Can you work these out from the drawing? Everything is in mm from the part's minimum corner. A direction names the side the tool comes from. Round coordinates to 2 decimals unless told otherwise and drop trailing zeros. Loops run counter-clockwise (first coordinate to the right, second up) from the corner with the lowest first, then second, coordinate; pieces in that order, holes last. Notation, with made-up numbers: M 15,86 L 51,86 A22 cw 51,104 Z; hole C 52,17.5 d3. An arc over 180 degrees is marked long. Answer in a Markdown table with one row per item.
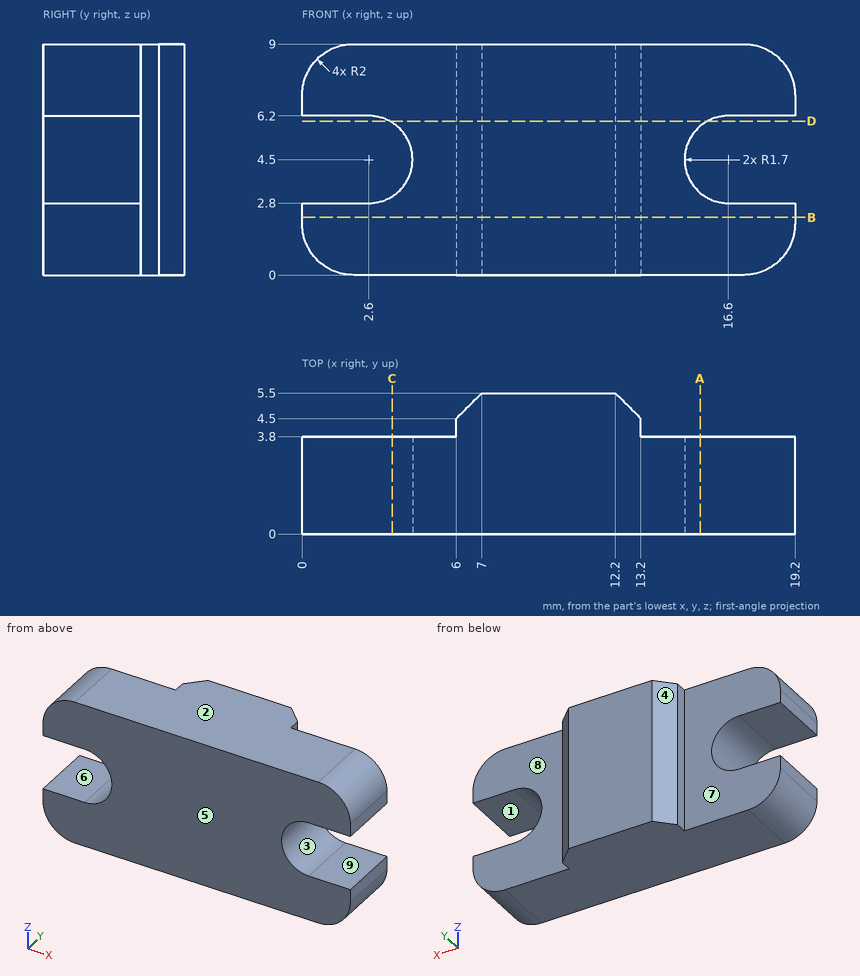
1) Will these pins go through, and if not, where does the flat tip stop? P1, Ø1, axis at x = 6, z = 7, coming from the +Y side; P2, Ø3, axis at x = 18, y = 1, coming from the -Z side; P3, Ø5, axis at x = 2.5, z = 4.5, coming from the +Y side; P4, Ø0.6, axis at y = 4, z = 4.5, coming from the +X side.
Computed:
| item | result |
|---|---|
| P1 | stops at y = 5 |
| P2 | stops at z = 0 |
| P3 | stops at y = 3.8 |
| P4 | stops at x = 14.91 |
2) I want a section at A-A, the plane x = 15.5. Please give me the cut outline in (y, z).
Computed:
| item | result |
|---|---|
| outline | M 0,0 L 3.8,0 L 3.8,3.2 L 0,3.2 Z; M 0,5.8 L 3.8,5.8 L 3.8,9 L 0,9 Z |
3) If we mould it in two halves opening along Z, with no side actions, what happens to the marked faces 1, 2, 3 and 4? For each: released by +Z, released by -Z, zero draft, split by the parting line, or undercut.
Computed:
| item | result |
|---|---|
| face 1 | undercut |
| face 2 | released by +Z |
| face 3 | undercut |
| face 4 | zero draft |
4) I want a section at B-B, the plane z = 2.25. Please give me the cut outline in (x, y).
Computed:
| item | result |
|---|---|
| outline | M 0,0 L 19.2,0 L 19.2,3.8 L 13.2,3.8 L 13.2,4.5 L 12.2,5.5 L 7,5.5 L 6,4.5 L 6,3.8 L 0,3.8 Z |
5) I need wall thicknesses on line 1 (Z direction, x = 2, y = 0.6); line 2 (X direction, y = 1.15, z = 4.5); line 3 (Y direction, x = 18.5, z = 1.5). Which ranges of each line are inside material? Lowest first, please.
Computed:
| item | result |
|---|---|
| line 1 | z = 0 to 2.8, 6.2 to 9 |
| line 2 | x = 4.3 to 14.9 |
| line 3 | y = 0 to 3.8 |
6) I want a section at C-C, the plane x = 3.5. Please give me the cut outline in (y, z).
Computed:
| item | result |
|---|---|
| outline | M 0,0 L 3.8,0 L 3.8,3.06 L 0,3.06 Z; M 0,5.94 L 3.8,5.94 L 3.8,9 L 0,9 Z |
7) Which directions (+Z, -Z, +X, -X, +Y, -Y) give clear straight access to the entire face, cutting with the end or side of a thin tool? Please do the marked faces 5, 6, 7, 8 and 9.
Computed:
| item | result |
|---|---|
| face 5 | +Z, -Z, +X, -X, -Y |
| face 6 | -X, +Y, -Y |
| face 7 | +Z, -Z, -X, +Y |
| face 8 | +Z, -Z, +X, +Y |
| face 9 | +X, +Y, -Y |
8) I want a section at D-D, the plane z = 6. Please give me the cut outline in (x, y).
Computed:
| item | result |
|---|---|
| outline | M 3.4,0 L 15.8,0 L 15.8,3.8 L 13.2,3.8 L 13.2,4.5 L 12.2,5.5 L 7,5.5 L 6,4.5 L 6,3.8 L 3.4,3.8 Z |
